Verification items for the finished model (mm, model axes). Give positions to 0.01 mm unless a question says otherwise; leave off trailing zeros. Write each loop counter-clockwise with the first axis right and the second up, starting at its lowest first coordinate (ties: lowest second). Pieces come first, ordered by that corner, then holes. Notation, with made-up numbers: (7.25, 37) - (39.25, 37) arc R23 cw to (39.25, 65) - close; hole circle Ø1 at (83.5, -7.75). An arc over 180 degrees is marked (long way). Answer as a JSON object with one key per item and string values. Group by question number.
Item 1: Sectioned sample at A-A, the plane z = 0. Record the boundary of the cut face in (x, y) (3 decimals).
Item 2: Sectioned sample at C-C, the plane z = 1.5. Record the boundary of the cut face in (x, y).
Item 3: Scan lines: line 1 along X through (y, z) = (3.75, 0); line 2 along Z through (x, y) = (0.79, 6.75); line 3 along Z through (x, y) = (0.79, 4.75). Record each from-to range of solid material in increasing order. Write a range as [from, to].
Item 4: Go/stop test with flat-tipped pins: pin 1 (4 mm diameter, centred on x = 2.5, y = 2.5, fed in from +Z); pin 2 (2 mm diameter, centred on x = -2.5, y = 4, fed in from +Z). Record where each tip stops, or that it passes through.
Item 5: Sectioned sample at B-B, the plane y = 1.75. Record the boundary of the cut face in (x, z), and give its area (3 significant figures).
```python
from build123d import *

# Parameters (mm, degrees)
BOSS_EXTRUDE1_DEPTH = 6
SKETCH2_R           = 3.555
BOSS_EXTRUDE2_DEPTH = 2.5
SKETCH3_R           = 2.5
CUT_EXTRUDE1_DEPTH  = 9.5
FILLET1_R           = 0.5


with BuildPart() as part:
    # Sketch1 → Boss-Extrude1 (new body)
    with BuildSketch(Plane(origin=(0, 0, 0), x_dir=(1, 0, 0), z_dir=(0, 1, 0))):
        Polygon((5, -2.886751346), (5, 2.886751346), (0, 5.773502692), (-5, 2.886751346), (-5, -2.886751346), (0, -5.773502692), align=None)
    extrude(amount=BOSS_EXTRUDE1_DEPTH)

    # Sketch2 → Boss-Extrude2 (add)
    with BuildSketch(Plane(origin=(0, 6, 0), x_dir=(1, 0, 0), z_dir=(0, 1, 0))):
        Circle(SKETCH2_R)
    extrude(amount=BOSS_EXTRUDE2_DEPTH)

    # Sketch3 → Cut-Extrude1 (cut, through all)
    with BuildSketch(Plane(origin=(0, 8.5, 0), x_dir=(1, 0, 0), z_dir=(0, 1, 0))):
        with Locations((0.79, 0)):
            Circle(SKETCH3_R)
    extrude(amount=-CUT_EXTRUDE1_DEPTH, mode=Mode.SUBTRACT)

    # Fillet1
    fillet1_edges = [part.edges().sort_by_distance(p)[0] for p in [
        (2.5, 6, -4.330127019),
        (-2.5, 6, -4.330127019),
        (-5, 6, 0),
        (-2.5, 6, 4.330127019),
        (2.5, 6, 4.330127019),
        (-2.5, 0, 4.330127019),
        (-5, 0, 0),
        (-2.5, 0, -4.330127019),
        (2.5, 0, -4.330127019),
        (5, 0, 0),
        (2.5, 0, 4.330127019),
        (5, 6, 0),
    ]]
    fillet(fillet1_edges, radius=FILLET1_R)


solid = part.part
```
Geometry check:
{
 "1": {"outline": "(-5, 0.5) arc R0.5 ccw to (-4.5, 0) - (-1.71, 0) - (-1.71, 8.5) - (-3.555, 8.5) - (-3.555, 6) - (-4.5, 6) arc R0.5 ccw to (-5, 5.5) - close; (3.29, 0) - (4.5, 0) arc R0.5 ccw to (5, 0.5) - (5, 5.5) arc R0.5 ccw to (4.5, 6) - (3.555, 6) - (3.555, 8.5) - (3.29, 8.5) - close"},
 "2": {"outline": "(-5, 0.5) arc R0.5 ccw to (-4.5, 0) - (-1.21, 0) - (-1.21, 8.5) - (-3.22, 8.5) - (-3.22, 6) - (-4.5, 6) arc R0.5 ccw to (-5, 5.5) - close; (2.79, 0) - (4.5, 0) arc R0.5 ccw to (5, 0.5) - (5, 5.5) arc R0.5 ccw to (4.5, 6) - (3.22, 6) - (3.22, 8.5) - (2.79, 8.5) - close"},
 "3": {"line 1": "[-5, -1.71], [3.29, 5]", "line 2": "[-3.47, -2.5], [2.5, 3.47]", "line 3": "[-5.32, -2.5], [2.5, 5.32]"},
 "4": {"pin 1": "z = 5.48", "pin 2": "z = 4.91"},
 "5": {"outline": "(-5, -2.89) - (0, -5.77) - (5, -2.89) - (5, 2.89) - (0, 5.77) - (-5, 2.89) - close; hole circle Ø5 at (0.79, 0)", "area": "67.0 mm^2"}
}
